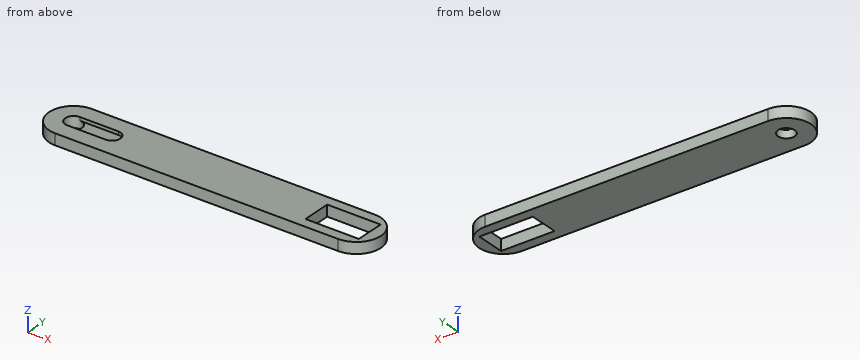
```python
from build123d import *

# Parameters (mm, degrees)
SKETCH1_R           = 3.75
SKETCH1_W           = 24
SKETCH1_H           = 13
BOSS_EXTRUDE1_DEPTH = 5
CUT_EXTRUDE1_DEPTH  = 1.5


with BuildPart() as part:
    # Sketch1 → Boss-Extrude1 (new body)
    with BuildSketch(Plane.XY):
        with BuildLine():
            ThreePointArc((0, 22), (-11, 11), (0, 0))
            Line((0, 0), (127, 0))
            ThreePointArc((127, 0), (138, 11), (127, 22))
            Line((127, 22), (0, 22))
        make_face()
        with Locations((0, 11)):
            Circle(SKETCH1_R, mode=Mode.SUBTRACT)
        with Locations((121, 11)):
            Rectangle(SKETCH1_W, SKETCH1_H, mode=Mode.SUBTRACT)
    extrude(amount=BOSS_EXTRUDE1_DEPTH)

    # Sketch3 → Cut-Extrude1 (cut)
    with BuildSketch(Plane.XY.offset(5)):
        with BuildLine():
            Line((0, 14.75), (17.25, 14.75))
            ThreePointArc((17.25, 14.75), (21, 11), (17.25, 7.25))
            Line((17.25, 7.25), (0, 7.25))
            ThreePointArc((0, 7.25), (3.75, 11), (0, 14.75))
        make_face()
    extrude(amount=-CUT_EXTRUDE1_DEPTH, mode=Mode.SUBTRACT)


solid = part.part
```
CAD build for the part. Positions are in the model's coordinates, mm. Give positions to 0.01 mm unless a question says otherwise; leave off trailing zeros. Write each loop counter-clockwise with the first axis right and the second up, starting at its lowest first coordinate (ties: lowest second). Pieces come first, ordered by that corner, then holes. Notation, with made-up numbers: M 16,-11.5 L 42,-11.5 A28 cw 42,23.5 Z; hole C -22,21 d11. An arc over 180 degrees is marked long. Return JSON: item names as keys, results as strings. Group by question number.
(1) Drill centre lines: L1, parallel to X at y = 11, z = 3.65; L2, parallel to X at y = 11, z = 2.15; L3, parallel to Y at x = 117.5, z = 2.95. Where is each one in solid material? Low to high. Write a range as [from, to].
(2) Flat gauge pins, fed straight in: pin 1 Ø1 at (x, z) = (30.5, 1.5) entering from -Y; pin 2 Ø2 at (x, y) = (7, 12) entering from +Z. Where does each tip first touch, or does it go through?
(3) Band-saw the part on C-C (z = 2.3). Give the cut face in (x, y), and give its area (3 significant figures).
(4) Band-saw the part on D-D (x = 6). Give the cut face in (y, z).
(5) Band-saw the part on A-A (y = 11). Give the cut face in (x, z), and give its area (3 significant figures).
(6) Band-saw the part on B-B (x = 112). Give the cut face in (y, z), and give its area (3 significant figures).
Entries:
{
 "1": {"L1": "x = [-11, -3.75], [21, 109], [133, 138]", "L2": "x = [-11, -3.75], [3.75, 109], [133, 138]", "L3": "y = [0, 4.5], [17.5, 22]"},
 "2": {"pin 1": "stops at y = 0", "pin 2": "stops at z = 3.5"},
 "3": {"outline": "M 0,0 L 127,0 A11 ccw 127,22 L 0,22 A11 ccw Z; hole C 0,11 d7.5; hole M 109,4.5 L 133,4.5 L 133,17.5 L 109,17.5 Z", "area": "2,820 mm^2"},
 "4": {"outline": "M 0,0 L 22,0 L 22,5 L 14.75,5 L 14.75,3.5 L 7.25,3.5 L 7.25,5 L 0,5 Z"},
 "5": {"outline": "M -11,0 L -3.75,0 L -3.75,5 L -11,5 Z; M 3.75,0 L 109,0 L 109,5 L 21,5 L 21,3.5 L 3.75,3.5 Z; M 133,0 L 138,0 L 138,5 L 133,5 Z", "area": "562 mm^2"},
 "6": {"outline": "M 0,0 L 4.5,0 L 4.5,5 L 0,5 Z; M 17.5,0 L 22,0 L 22,5 L 17.5,5 Z", "area": "45.0 mm^2"}
}
